Part model, mm, in its own coordinate system. A direction names the side the tool comes from. Round coordinates to 2 decimals unless told otherwise and drop trailing zeros. Loops run counter-clockwise (first coordinate to the right, second up) from the corner with the lowest first, then second, coordinate; pieces in that order, holes last. Notation, with made-up numbers: (41, 22) -> (78, 22) arc R23 cw to (78, 54) -> close; hole circle Ø6 at (86, 43). An arc over 180 degrees is marked (long way). Use a Markdown table: item, result. Add a question column.
Item 1: Cut at A-A, the plane y = 0. List the corners of the cut face in (x, z) (3 decimals).
Item 2: Which spindle directions (+Z, -Z, +X, -X, +Y, -Y) get a long thin tool onto all of the face, cutting with end or side? Do faces 1 (the face through (0, 0, 0)), 2 (the face through (-2.13, -1.914, -0.251)), 3 (the face through (-32.17, -0.46, 1.47)). Say none if no direction does.
Item 3: Cut at D-D, the plane x = -20. List the corners of the cut face in (y, z).
Item 4: Flat gauge pins, fed straight in: pin 1 (1 mm diameter, centred on x = -15.5, y = 2, fed in from +Z); pin 2 (2 mm diameter, centred on x = -43.5, y = -0.5, fed in from +Z); pin 3 (3 mm diameter, centred on x = -24, z = 1, fed in from +Y). Where does each tip first touch, or does it go through?
Item 5: Probe line 1 (Z direction, x = -6.5, y = -0.25); line 2 (X direction, y = 1.65, z = -1.4); line 3 (Y direction, x = -28.5, z = -1.4). List the from-to ranges inside material, lowest first. Write a range as [from, to].
Item 6: Cut at C-C, the plane x = -10.5. List the corners of the cut face in (y, z), plus the area to 3 significant figures.
```python
from build123d import *

# Parameters (mm, degrees)
F4_R     = 0.762
F5_SIZE2 = 0.3287820151
F5_SIZE  = 0.79375


# Not quite as in the source:
# - a fillet or chamfer that OpenCascade refuses, or shapes differently, is made with other operations: its cross-section is extruded or revolved along the edge and cut away or added


with BuildPart() as f1:
    # F0 (on Front) → F1 (revolve)
    with BuildSketch(Plane.XZ):
        with BuildLine():
            Line((-58.3184, 0), (0, 0))
            Line((0, 0), (0, 1.9304))
            Line((0, 1.9304), (-4.191, 1.9304))
            Line((-4.191, 1.9304), (-4.191, 2.7432))
            Line((-4.191, 2.7432), (-8.382, 2.7432))
            Line((-8.382, 2.7432), (-8.382, 2.54))
            Line((-8.382, 2.54), (-18.415, 2.54))
            Line((-18.415, 2.54), (-18.415, 1.9431))
            Line((-18.415, 1.9431), (-45.2374, 1.1557))
            Line((-45.2374, 1.1557), (-57.1627, 1.1557))
            ThreePointArc((-57.1627, 1.1557), (-57.979903307, 0.817203307), (-58.3184, 0))
        make_face()
    revolve(axis=Axis((-29.1592, 0, 0), (1, 0, 0)))

    # F2: fillet of radius 3.175 on 1 edges, made by hand

    # F2_s1 → F2_t2 (revolve)
    with BuildSketch(Plane.XZ):
        with BuildLine():
            ThreePointArc((-45.1908273531, 1.1570671894), (-45.2374050161, 1.1560418158), (-45.2839927102, 1.1557))
            Line((-45.2839927102, 1.1557), (-45.2374, 1.1557))
            Line((-45.2374, 1.1557), (-45.1908273531, 1.1570671894))
        make_face()
    revolve(axis=Axis((-45.2374, 0, 0), (1, 0, 0)))

    # F3: fillet of radius 0.381 on 2 edges, made by hand

    # F3_s1 → F3_t2 (revolve)
    with BuildSketch(Plane.XZ):
        with BuildLine():
            ThreePointArc((-18.7848201571, 1.9322435371), (-18.5226682235, 2.0476538916), (-18.415, 2.3130794743))
            Line((-18.415, 2.3130794743), (-18.40738, 2.3130794743))
            Line((-18.40738, 2.3130794743), (-18.40738, 1.9357004105))
            Line((-18.40738, 1.9357004105), (-18.7845965603, 1.9246268183))
            Line((-18.7845965603, 1.9246268183), (-18.7848201571, 1.9322435371))
        make_face()
    revolve(axis=Axis((-18.415, 0, 0), (1, 0, 0)))

    # F3_s3 → F3_t4 (revolve)
    with BuildSketch(Plane.XZ):
        with BuildLine():
            ThreePointArc((-8.7189690787, 2.54), (-8.5222215247, 2.5947310925), (-8.382, 2.7432))
            Line((-8.382, 2.7432), (-8.3752606184, 2.739644))
            ThreePointArc((-8.3752606184, 2.739644), (-8.37438, 2.6416), (-8.37438, 2.54))
            Line((-8.37438, 2.54), (-8.382, 2.53238))
            Line((-8.382, 2.53238), (-8.7189690787, 2.53238))
            Line((-8.7189690787, 2.53238), (-8.7189690787, 2.54))
        make_face()
    revolve(axis=Axis((-8.382, 0, 0), (1, 0, 0)))

    # F4
    f4_edges = [f1.edges().sort_by_distance(p)[0] for p in [
        (-4.191, 0, -1.9304),
    ]]
    fillet(f4_edges, radius=F4_R)

    # F5
    f5_edges = [f1.edges().sort_by_distance(p)[0] for p in [
        (0, 0, -1.9304),
    ]]
    chamfer(f5_edges, length=F5_SIZE, length2=F5_SIZE2)


solid = f1.part
```
A:
| question | item | result |
|---|---|---|
| 1 | outline | (-57.163, -1.156) -> (-45.284, -1.156) arc R3.175 cw to (-45.191, -1.157) -> (-18.785, -1.932) arc R0.381 cw to (-18.415, -2.313) -> (-18.415, -2.54) -> (-8.719, -2.54) arc R0.381 cw to (-8.382, -2.743) -> (-4.191, -2.743) -> (-4.191, -2.692) arc R0.762 cw to (-3.429, -1.93) -> (-0.794, -1.93) -> (0, -1.602) -> (0, 1.602) -> (-0.794, 1.93) -> (-3.429, 1.93) arc R0.762 cw to (-4.191, 2.692) -> (-4.191, 2.743) -> (-8.382, 2.743) arc R0.381 cw to (-8.719, 2.54) -> (-18.415, 2.54) -> (-18.415, 2.313) arc R0.381 cw to (-18.785, 1.932) -> (-45.191, 1.157) arc R3.175 cw to (-45.284, 1.156) -> (-57.163, 1.156) arc R1.156 ccw to start |
| 2 | face 1 | +Z, -Z, +X, +Y, -Y |
| 2 | face 2 | +X |
| 2 | face 3 | -X |
| 3 | outline | circle Ø3.79 at (0, 0) |
| 4 | pin 1 | stops at z = 2.05 |
| 4 | pin 2 | stops at z = 1.23 |
| 4 | pin 3 | stops at y = 1.81 |
| 5 | line 1 | z = [-2.73, 2.73] |
| 5 | line 2 | x = [-18.45, -3.98] |
| 5 | line 3 | y = [-0.87, 0.87] |
| 6 | outline | circle Ø5.08 at (0, 0) |
| 6 | area | 20.3 mm^2 |
